Check sheet for the modelled part. Datum: model origin and axes. Units: mm. Face numbers are marked on the shaded views. A direction names the side the tool comes from. Give positions to 0.01 mm unless a question says otherwise; leave off trailing zeros. Write each loop counter-clockwise with the first axis right and the second up, starting at its lowest first coordinate (ties: lowest second). Pieces come first, ordered by that corner, then holes. Notation, with made-up numbers: (3.25, 89.5) -> (46.25, 89.5) arc R19 ccw to (46.25, 114.5) -> close; hole circle Ø7 at (-27.5, 40). An arc over 180 degrees is marked (long way). Write each question's results on one line, items separated by ' | '. Start each with the question number.
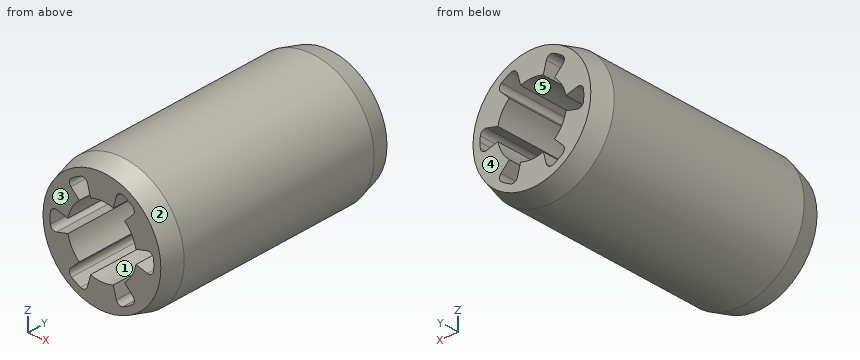
```python
from build123d import *

# Parameters (mm, degrees)
F0_R     = 6.5
F1_DEPTH = 25
F2_R     = 0.5
F3_SIZE2 = 0.5358983849
F3_SIZE  = 2


with BuildPart() as f1:
    # F0 (on Front) → F1 (new body)
    with BuildSketch(Plane.XZ):
        Circle(F0_R)
        with BuildLine():
            ThreePointArc((5.1311754503, 1.1106477833), (5.2202093403, 0.5584930108), (5.25, 0))
            ThreePointArc((5.25, 0), (5.2202093403, -0.5584930108), (5.1311754503, -1.1106477833))
            ThreePointArc((5.1311754503, -1.1106477833), (4.5466333699, -2.625), (3.5274369202, -3.8884043995))
            ThreePointArc((3.5274369202, -3.8884043995), (2.625, -4.5466333699), (1.6037385301, -4.9990521829))
            ThreePointArc((1.6037385301, -4.9990521829), (0, -5.25), (-1.6037385301, -4.9990521829))
            ThreePointArc((-1.6037385301, -4.9990521829), (-2.625, -4.5466333699), (-3.5274369202, -3.8884043995))
            ThreePointArc((-3.5274369202, -3.8884043995), (-4.5466333699, -2.625), (-5.1311754503, -1.1106477833))
            ThreePointArc((-5.1311754503, -1.1106477833), (-5.25, 0), (-5.1311754503, 1.1106477833))
            ThreePointArc((-5.1311754503, 1.1106477833), (-4.5466333699, 2.625), (-3.5274369202, 3.8884043995))
            ThreePointArc((-3.5274369202, 3.8884043995), (-2.625, 4.5466333699), (-1.6037385301, 4.9990521829))
            ThreePointArc((-1.6037385301, 4.9990521829), (0, 5.25), (1.6037385301, 4.9990521829))
            ThreePointArc((1.6037385301, 4.9990521829), (2.625, 4.5466333699), (3.5274369202, 3.8884043995))
            ThreePointArc((3.5274369202, 3.8884043995), (4.5466333699, 2.625), (5.1311754503, 1.1106477833))
        make_face(mode=Mode.SUBTRACT)
        with BuildLine():
            Line((1.15, 3.3056769352), (1.6037385301, 4.9990521829))
            ThreePointArc((1.6037385301, 4.9990521829), (0, 5.25), (-1.6037385301, 4.9990521829))
            Line((-1.6037385301, 4.9990521829), (-1.15, 3.3056769352))
            ThreePointArc((-1.15, 3.3056769352), (0, 3.5), (1.15, 3.3056769352))
        make_face()
        with BuildLine():
            Line((3.4378002026, 0.6569092533), (5.1311754503, 1.1106477833))
            ThreePointArc((5.1311754503, 1.1106477833), (4.5466333699, 2.625), (3.5274369202, 3.8884043995))
            Line((3.5274369202, 3.8884043995), (2.2878002026, 2.648767682))
            ThreePointArc((2.2878002026, 2.648767682), (3.0310889132, 1.75), (3.4378002026, 0.6569092533))
        make_face()
        with BuildLine():
            ThreePointArc((3.5274369202, -3.8884043995), (4.5466333699, -2.625), (5.1311754503, -1.1106477833))
            Line((5.1311754503, -1.1106477833), (3.4378002026, -0.6569092533))
            ThreePointArc((3.4378002026, -0.6569092533), (3.0310889132, -1.75), (2.2878002026, -2.648767682))
            Line((2.2878002026, -2.648767682), (3.5274369202, -3.8884043995))
        make_face()
        with BuildLine():
            ThreePointArc((-1.6037385301, -4.9990521829), (0, -5.25), (1.6037385301, -4.9990521829))
            Line((1.6037385301, -4.9990521829), (1.15, -3.3056769352))
            ThreePointArc((1.15, -3.3056769352), (0, -3.5), (-1.15, -3.3056769352))
            Line((-1.15, -3.3056769352), (-1.6037385301, -4.9990521829))
        make_face()
        with BuildLine():
            ThreePointArc((-5.1311754503, -1.1106477833), (-4.5466333699, -2.625), (-3.5274369202, -3.8884043995))
            Line((-3.5274369202, -3.8884043995), (-2.2878002026, -2.648767682))
            ThreePointArc((-2.2878002026, -2.648767682), (-3.0310889132, -1.75), (-3.4378002026, -0.6569092533))
            Line((-3.4378002026, -0.6569092533), (-5.1311754503, -1.1106477833))
        make_face()
        with BuildLine():
            Line((-2.2878002026, 2.648767682), (-3.5274369202, 3.8884043995))
            ThreePointArc((-3.5274369202, 3.8884043995), (-4.5466333699, 2.625), (-5.1311754503, 1.1106477833))
            Line((-5.1311754503, 1.1106477833), (-3.4378002026, 0.6569092533))
            ThreePointArc((-3.4378002026, 0.6569092533), (-3.0310889132, 1.75), (-2.2878002026, 2.648767682))
        make_face()
    extrude(amount=F1_DEPTH)

    # F2
    f2_edges = [f1.edges().sort_by_distance(p)[0] for p in [
        (-3.527437, -12.5, 3.888404),
        (-1.603739, -12.5, 4.999052),
        (1.603739, -12.5, 4.999052),
        (3.527437, -12.5, 3.888404),
        (5.131175, -12.5, 1.110648),
        (5.131175, -12.5, -1.110648),
        (3.527437, -12.5, -3.888404),
        (1.603739, -12.5, -4.999052),
        (-1.603739, -12.5, -4.999052),
        (-3.527437, -12.5, -3.888404),
        (-5.131175, -12.5, -1.110648),
        (-5.131175, -12.5, 1.110648),
    ]]
    fillet(f2_edges, radius=F2_R)

    # F3
    f3_edges = [f1.edges().sort_by_distance(p)[0] for p in [
        (6.5, -12.5, 0),
        (-6.5, 0, 0),
        (-6.5, -25, 0),
    ]]
    f3_side = f1.faces().sort_by_distance((-6.5, -12.5, 0))[0]
    chamfer(f3_edges, length=F3_SIZE, length2=F3_SIZE2, reference=f3_side)


solid = f1.part
```
Item 1: Set-up check for the marked faces 4 and 5: record each of +Z, -Z, +X, -X, +Y, -Y from which the full face is reachable in a straight line by a thin tool's end or side.
Item 2: Thickness scan on probe 1 along Z at (x, y) = (2.5, -11.75); probe 2 along X at (y, z) = (-20.5, 3.75); probe 3 along Z at (x, y) = (-0.25, -21). Record the ranges inside material, lowest first. Write a range as from..to.
Item 3: Mould release check, pull along X, two halves, no side actions. Record for the marked faces 1, 2 and 3: pulls with the +X half, pulls with the -X half, needs draft (parallel to the pull), parting line crosses it, or undercut.
Item 4: Section check B-B on x = -2.75. Count the separate pieces of the cut face and the enclosed holes in it, then the cut area to 3 significant figures.
Item 5: Section check A-A on x = 0. Record the boundary of the cut face in (y, z).
Check sheet entries:
1) face 4: +Z, -Z, +X, -X, +Y | face 5: +Y, -Y
2) probe 1: z = -6..-4.62, -2.86..-2.45, 2.45..2.86, 4.62..6 | probe 2: x = -5.31..-3.27, -1.27..1.27, 3.27..5.31 | probe 3: z = -6.5..-3.49, 3.49..6.5
3) face 1: undercut | face 2: parting line crosses it | face 3: needs draft
4) separate pieces: 4 | enclosed holes: 0 | area: 116 mm^2
5) outline: (-25, -5.96) -> (-23, -6.5) -> (-2, -6.5) -> (0, -5.96) -> (0, -3.5) -> (-25, -3.5) -> close; (-25, 3.5) -> (0, 3.5) -> (0, 5.96) -> (-2, 6.5) -> (-23, 6.5) -> (-25, 5.96) -> close
